Study the drawing (mm; zero at the part's minimum x, y, z) and answer. Coordinates: 2 decimals unless noted, no trailing zeros. Order: outer loops, then holes, each group sorted by start corner. A loop starts at its lowest first (then second) coordinate and runs counter-clockwise, first axis right, second up. Notation, with made-up numbers: M 85,39.25 L 110,39.25 A37 ccw 110,76.25 Z; hole C 52,63.25 d7. An arc over 180 degrees is marked long. Use a Markdown table: item, result. Add a question column.
1) Find the intervals of material crossed by probe 1 along X at (y, z) = (56, 2.2); probe 2 along Y at (x, z) = (44.45, 0.8) (1 decimal); probe 3 along Y at (x, z) = (32, 2.9) (3 decimals), in increasing order. Write a range as [from, to].
2) Find section A-A on x = 31.75. Write down the section's boundary in (y, z) (1 decimal).
3) Find section B-B on y = 5.08. Count the separate pieces of the cut face and the enclosed holes in it, plus the area to 3 significant figures.
4) Find section D-D on y = 42. Write down the section's boundary in (x, z) (3 decimals), plus the area to 3 significant figures.
5) This flat-tipped pin is pushed along its axis until it touches: pin 1 Ø1 at (x, z) = (17.5, 2) entering from -Y (3 decimals). Where does it stop, or does it pass through?
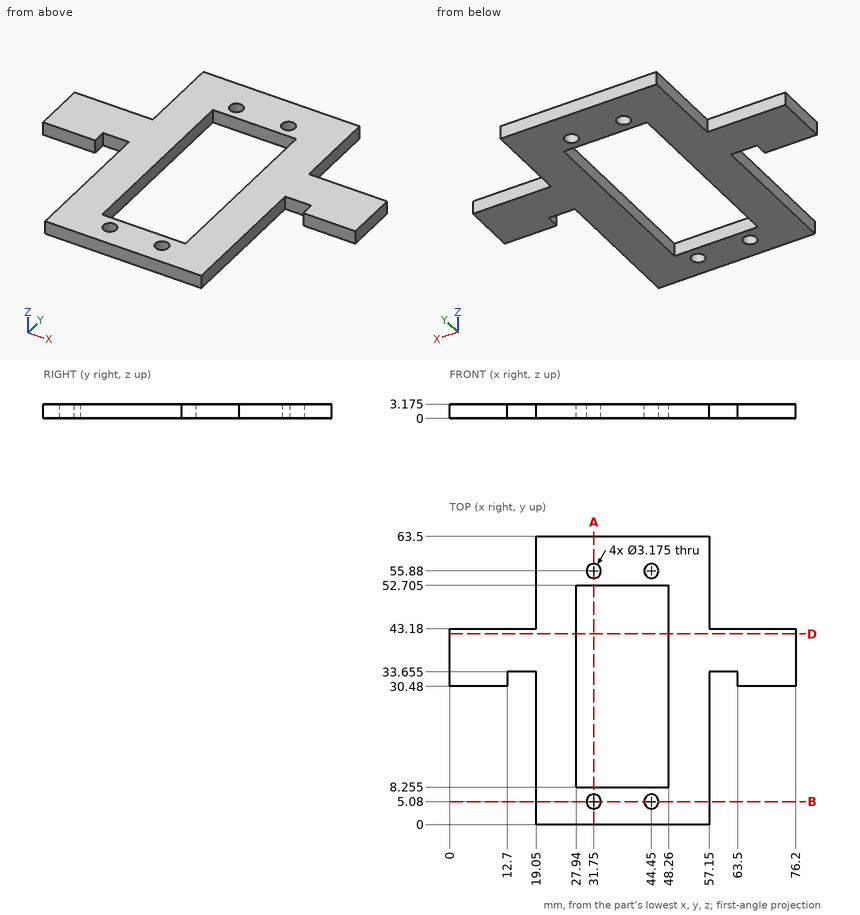
Check result:
| question | item | result |
|---|---|---|
| 1 | probe 1 | x = [19.05, 30.17], [33.33, 42.87], [46.03, 57.15] |
| 1 | probe 2 | y = [0, 3.5], [6.7, 8.3], [52.7, 54.3], [57.5, 63.5] |
| 1 | probe 3 | y = [0, 3.512], [6.648, 8.255], [52.705, 54.312], [57.448, 63.5] |
| 2 | outline | M 0,0 L 3.5,0 L 3.5,3.2 L 0,3.2 Z; M 6.7,0 L 8.3,0 L 8.3,3.2 L 6.7,3.2 Z; M 52.7,0 L 54.3,0 L 54.3,3.2 L 52.7,3.2 Z; M 57.5,0 L 63.5,0 L 63.5,3.2 L 57.5,3.2 Z |
| 3 | separate pieces | 3 |
| 3 | enclosed holes | 0 |
| 3 | area | 101 mm2 |
| 4 | outline | M 0,0 L 27.94,0 L 27.94,3.175 L 0,3.175 Z; M 48.26,0 L 76.2,0 L 76.2,3.175 L 48.26,3.175 Z |
| 4 | area | 177 mm2 |
| 5 | pin 1 | stops at y = 33.655 |
